```python
from build123d import *

# Parameters (mm, degrees)
F0_R     = 1.55
F0_W     = 52.2
F0_H     = 52.2
F0_W_2   = 10
F0_H_2   = 10
F0_R_2   = 10.5
F1_DEPTH = 4


with BuildPart() as f1:
    # F0 (on Top) → F1 (new body)
    with BuildSketch(Plane.XY):
        Polygon((10, 10), (10, 0), (105, 0), (105, 10), (115, 10), (115, 0), (210, 0), (210, 10), (220, 10), (220, 125), (210, 125), (210, 135), (220, 135), (220, 250), (210, 250), (210, 260), (115, 260), (115, 250), (105, 250), (105, 260), (10, 260), (10, 250), (0, 250), (0, 135), (10, 135), (10, 125), (0, 125), (0, 10), align=None)
        with Locations((16.561597, 30.703403)):
            Circle(F0_R, mode=Mode.SUBTRACT)
        with Locations((37.265, 10)):
            Circle(F0_R, mode=Mode.SUBTRACT)
        with Locations((30.703403, 16.561597)):
            Circle(F0_R, mode=Mode.SUBTRACT)
        with Locations((10, 37.265)):
            Circle(F0_R, mode=Mode.SUBTRACT)
        with Locations((67.265, 10)):
            Circle(F0_R, mode=Mode.SUBTRACT)
        with Locations((100, 5)):
            Circle(F0_R, mode=Mode.SUBTRACT)
        with Locations((78.9, 55)):
            Circle(F0_R, mode=Mode.SUBTRACT)
        with Locations((10, 67.265)):
            Circle(F0_R, mode=Mode.SUBTRACT)
        with Locations((152.735, 10)):
            Circle(F0_R, mode=Mode.SUBTRACT)
        with Locations((110, 55)):
            Rectangle(F0_W, F0_H, mode=Mode.SUBTRACT)
        with Locations((141.1, 55)):
            Circle(F0_R, mode=Mode.SUBTRACT)
        with Locations((182.735, 10)):
            Circle(F0_R, mode=Mode.SUBTRACT)
        with Locations((189.296597, 16.561597)):
            Circle(F0_R, mode=Mode.SUBTRACT)
        with Locations((203.438403, 30.703403)):
            Circle(F0_R, mode=Mode.SUBTRACT)
        with Locations((210, 37.265)):
            Circle(F0_R, mode=Mode.SUBTRACT)
        with Locations((110, 86.1)):
            Circle(F0_R, mode=Mode.SUBTRACT)
        with Locations((110, 110.7335)):
            Rectangle(F0_W_2, F0_H_2, mode=Mode.SUBTRACT)
        with Locations((110, 123.2335)):
            Circle(F0_R, mode=Mode.SUBTRACT)
        with Locations((210, 67.265)):
            Circle(F0_R, mode=Mode.SUBTRACT)
        with Locations((215, 120)):
            Circle(F0_R, mode=Mode.SUBTRACT)
        with Locations((5, 140)):
            Circle(F0_R, mode=Mode.SUBTRACT)
        with Locations((10, 192.735)):
            Circle(F0_R, mode=Mode.SUBTRACT)
        with Locations((80, 140.7335)):
            Rectangle(F0_W_2, F0_H_2, mode=Mode.SUBTRACT)
        with Locations((92.5, 140.7335)):
            Circle(F0_R, mode=Mode.SUBTRACT)
        with Locations((10, 222.735)):
            Circle(F0_R, mode=Mode.SUBTRACT)
        with Locations((16.561597, 229.296597)):
            Circle(F0_R, mode=Mode.SUBTRACT)
        with Locations((30.703403, 243.438403)):
            Circle(F0_R, mode=Mode.SUBTRACT)
        with Locations((37.265, 250)):
            Circle(F0_R, mode=Mode.SUBTRACT)
        with Locations((67.265, 250)):
            Circle(F0_R, mode=Mode.SUBTRACT)
        with Locations((110, 140.7335)):
            Circle(F0_R_2, mode=Mode.SUBTRACT)
        with Locations((127.5, 140.7335)):
            Circle(F0_R, mode=Mode.SUBTRACT)
        with Locations((110, 158.2335)):
            Circle(F0_R, mode=Mode.SUBTRACT)
        with Locations((140, 140.7335)):
            Rectangle(F0_W_2, F0_H_2, mode=Mode.SUBTRACT)
        with Locations((110, 170.7335)):
            Rectangle(F0_W_2, F0_H_2, mode=Mode.SUBTRACT)
        with Locations((210, 192.735)):
            Circle(F0_R, mode=Mode.SUBTRACT)
        with Locations((120, 255)):
            Circle(F0_R, mode=Mode.SUBTRACT)
        with Locations((152.735, 250)):
            Circle(F0_R, mode=Mode.SUBTRACT)
        with Locations((210, 222.735)):
            Circle(F0_R, mode=Mode.SUBTRACT)
        with Locations((189.296597, 243.438403)):
            Circle(F0_R, mode=Mode.SUBTRACT)
        with Locations((182.735, 250)):
            Circle(F0_R, mode=Mode.SUBTRACT)
        with Locations((203.438403, 229.296597)):
            Circle(F0_R, mode=Mode.SUBTRACT)
    extrude(amount=F1_DEPTH)


solid = f1.part
```
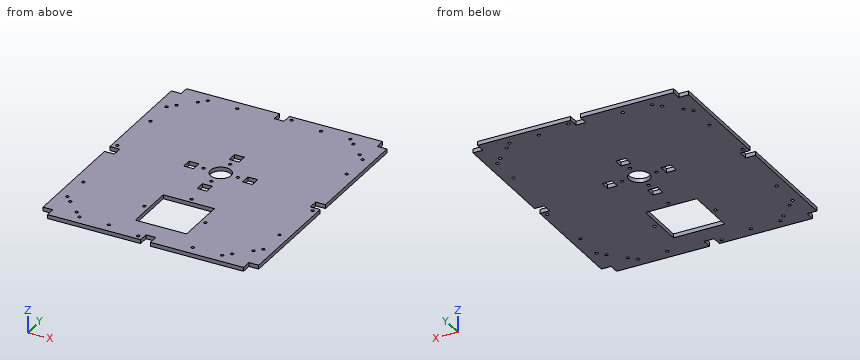
Source: CAD feature listing. Evaluate the final solid. Frame: model axes, mm. Give positions to 0.01 mm unless a question says otherwise; leave off trailing zeros. Order: outer loops, then holes, each group sorted by start corner. A loop starts at its lowest first (then second) coordinate and runs counter-clockwise, first axis right, second up.
(1) Contact query for flat-ended pins moving along their axis: P1, Ø1.2, axis at y = 129.5, z = 2.5, coming from the +X side; P2, Ø1.2, axis at y = 7.5, z = 2.5, coming from the -X side. Output: stop coordinate, or through.
(2) Section query B-B (y = 111). Return the cut outline in (x, z).
(3) Material intervals for line 1 along Y through (x, z) = (141.5, 3.6); line 2 along Y through (x, z) = (67.5, 3.3); line 3 along Y through (x, z) = (119.5, 1.35), sorted ascending.
(4) Section query C-C (z = 1.45). State how many separate pieces and enclosed holes the cut face has, plus the area to 3 significant figures.
(5) Section query A-A (y = 49.5). Return the cut outline in (x, z), plus the area to 3 significant figures.
Outcome:
1. P1: stops at x = 210
1. P2: stops at x = 10
2. outline: (0, 0) - (105, 0) - (105, 4) - (0, 4) - close; (115, 0) - (220, 0) - (220, 4) - (115, 4) - close
3. line 1: y = 0 to 53.5, 56.5 to 135.73, 145.73 to 260
3. line 2: y = 0 to 8.47, 11.53 to 248.47, 251.53 to 260
3. line 3: y = 0 to 28.9, 81.1 to 136.26, 145.21 to 253.53, 256.47 to 260
4. separate pieces: 1
4. enclosed holes: 41
4. area: 52,700 mm2
5. outline: (0, 0) - (83.9, 0) - (83.9, 4) - (0, 4) - close; (136.1, 0) - (220, 0) - (220, 4) - (136.1, 4) - close
5. area: 671 mm2
